from build123d import *

# Parameters (mm, degrees)
SKETCH_3_R          = 11.768421734
CUT_EXTRUDE_1_DEPTH = 10


with BuildPart() as part:
    # 草图1 → 旋转1 (revolve)
    with BuildSketch(Plane.XY, mode=Mode.PRIVATE) as revolve_1_sk:
        with BuildLine():
            Line((0, 0), (25, 0))
            Line((25, 0), (25, 3.134686744))
            ThreePointArc((25, 3.134686744), (24.76494299, 4.298770187), (24.096606492, 5.280436315))
            Line((24.096606492, 5.280436315), (12.874273498, 16.24574957))
            ThreePointArc((12.874273498, 16.24574957), (11.909645648, 16.878241234), (10.777667007, 17.1))
            Line((10.777667007, 17.1), (4, 17.1))
            Line((4, 17.1), (4, 25.1))
            Line((4, 25.1), (7.5, 25.1))
            Line((7.5, 25.1), (7.5, 33))
            Line((7.5, 33), (4, 33))
            Line((4, 33), (4, 83))
            Line((4, 83), (0, 83))
            Line((0, 83), (0, 0))
        make_face()
    revolve(revolve_1_sk.sketch.rotate(Axis((0, 83, 0), (0, 1, 0)), 270), axis=Axis((0, 83, 0), (0, 1, 0)))

    # 草图3 → 切除-拉伸1 (cut)
    with BuildSketch(Plane(origin=(0, 33, 0), x_dir=(1, 0, 0), z_dir=(0, 1, 0))):
        Circle(SKETCH_3_R)
        Polygon((7.5, 0), (3.75, 6.495190528), (-3.75, 6.495190528), (-7.5, 0), (-3.75, -6.495190528), (3.75, -6.495190528), align=None, mode=Mode.SUBTRACT)
    extrude(amount=-CUT_EXTRUDE_1_DEPTH, mode=Mode.SUBTRACT)


solid = part.part
Can you work these out from the model? Positions are in its coordinate system, mm. A direction names the side the tool comes from. Give positions to 0.01 mm unless a question says otherwise; leave off trailing zeros. Order: outer loops, then holes, each group sorted by start corner. A loop starts at its lowest first (then second) coordinate and runs counter-clockwise, first axis right, second up. Notation, with made-up numbers: M 38,-7 L 57,-7 A23 cw 57,25 Z; hole C 68.5,-21 d2. An arc over 180 degrees is marked long. Use one line per item in the form item = value. Start each with the question number.
Item 1: For faces 4 (the flat face through (0, 17.1, 5)), 5 (the flat face through (-5.6, 29.11, -3.29)), 6 (the flat face through (0, 29, -6.495)), 7 (the flat face through (0, 29, 6.495)), which set-ups out of +Z, -Z, +X, -X, +Y, -Y let a thin tool reach every point of the face, with its end or its side?
Item 2: Will these pins go through, and if not, where does the flat tip stop? pin 1 Ø8 at (x, y) = (-1, 28.5) entering from +Z; pin 2 Ø10 at (x, z) = (-15.5, 2) entering from +Y; pin 3 Ø2 at (x, y) = (1, 28) entering from -Z.
Item 3: We'd pull the mould along Y, two halves only. Please class faces 1 (the cylindrical face through (-3.905, 21.156, -0.867)), 2 (the cylindrical face through (-3.905, 58.35, -0.867)), 3 (the flat face through (0, 0, 0)): +Y half, -Y half, draft (parallel to the pull), parting line (faces both ways), or undercut.
Item 4: If I drill on line 1 along Y through (x, z) = (-5, -4); line 2 along Y through (x, z) = (9.5, 3); line 3 along Y through (x, z) = (-8, -16.5), over which ranges is the centre line in solid material (lowest first)?
Item 5: If we section it at B-B (y = 59): Write out the boundary of the cut face in (x, z), then the cut area to 3 significant figures.
Item 6: If we section it at A-A (x = 0): Write out the boundary of the cut face in (y, z), then the cut area to 3 significant figures.
Outcome:
q1.face_4 = none
q1.face_5 = -Z, -X, +Y
q1.face_6 = -Z, +X, -X, +Y
q1.face_7 = +Z, +X, -X, +Y
q2.pin_1 = 6.5
q2.pin_2 = 17.1
q2.pin_3 = -6.5
q3.face_1 = undercut
q3.face_2 = draft
q3.face_3 = -Y half
q4.line_1 = 0 to 17.1, 25.1 to 33
q4.line_2 = 0 to 17.1
q4.line_3 = 0 to 10.91
q5.outline = C 0,0 d8
q5.area = 50.3 mm2
q6.outline = M 0,-25 L 3.13,-25 A3 ccw 5.28,-24.1 L 16.25,-12.87 A3 ccw 17.1,-10.78 L 17.1,-4 L 25.1,-4 L 25.1,-6.5 L 33,-6.5 L 33,-4 L 83,-4 L 83,4 L 33,4 L 33,6.5 L 25.1,6.5 L 25.1,4 L 17.1,4 L 17.1,10.78 A3 ccw 16.25,12.87 L 5.28,24.1 A3 ccw 3.13,25 L 0,25 Z
q6.area = 1,260 mm2
